For this review, take the finished solid that the model builds, in its own axes (mm). Face numbers are marked on the shaded views. Give positions to 0.01 mm unless a question says otherwise; leave off trailing zeros. Write each loop counter-clockwise with the first axis right and the second up, starting at its lowest first coordinate (ties: lowest second). Pieces come first, ordered by that corner, then holes.
from build123d import *

# Parameters (mm, degrees)
SKETCH_1_W               = 4
SKETCH_1_H               = 2.4
SKETCH_2_OUTSIDE_W       = 12.314
SKETCH_2_OUTSIDE_H       = 12.314
CUT_EXTRUDE_1_DEPTH      = 2.4
SKETCH_3_R               = 1.5
CUT_EXTRUDE_2_DEPTH      = 1
CUT_EXTRUDE_2_DEPTH_BACK = 3.4
CHAMFER_1_SIZE           = 0.4


with BuildPart() as part:
    # Эскиз1 → Повернуть1 (revolve)
    with BuildSketch(Plane(origin=(0, 0, 0), x_dir=(1, 0, 0), z_dir=(0, 1, 0))):
        with Locations((-2, 1.2)):
            Rectangle(SKETCH_1_W, SKETCH_1_H)
    revolve(axis=Axis((0, 0, 0), (0, 0, -1)))

    # Эскиз2 outside → Вырез-Вытянуть1 (cut)
    with BuildSketch(Plane.XY):
        Rectangle(SKETCH_2_OUTSIDE_W, SKETCH_2_OUTSIDE_H)
        Polygon((2.75, -1.58771324), (2.75, 1.58771324), (0, 3.175426481), (-2.75, 1.58771324), (-2.75, -1.58771324), (0, -3.175426481), align=None, mode=Mode.SUBTRACT)
    extrude(amount=-CUT_EXTRUDE_1_DEPTH, mode=Mode.SUBTRACT)

    # Эскиз3 → Вырез-Вытянуть2 (cut, two sides)
    with BuildSketch(Plane.XY) as cut_extrude_2_sk:
        Circle(SKETCH_3_R)
    extrude(amount=CUT_EXTRUDE_2_DEPTH, mode=Mode.SUBTRACT)
    extrude(cut_extrude_2_sk.sketch, amount=-CUT_EXTRUDE_2_DEPTH_BACK, mode=Mode.SUBTRACT)

    # Эскиз4 → Вырез-Повернуть1 (revolve, cut)
    with BuildSketch(Plane(origin=(0, 0, 0), x_dir=(0, 0, -1), z_dir=(1, 0, 0))):
        Polygon((0, 2.6), (0.332222633, 3.175426481), (0, 3.175426481), align=None)
        Polygon((2.4, 2.6), (2.067777367, 3.175426481), (2.4, 3.175426481), align=None)
    revolve(axis=Axis((0, 0, 0), (0, 0, -1)), mode=Mode.SUBTRACT)

    # Фаска1
    chamfer_1_edges = [part.edges().sort_by_distance(p)[0] for p in [
        (-1.5, 0, -2.4),
        (-1.5, 0, 0),
    ]]
    chamfer(chamfer_1_edges, length=CHAMFER_1_SIZE)


solid = part.part
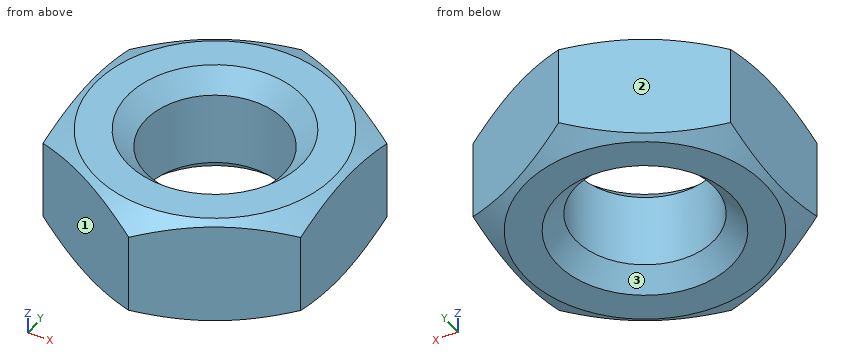
(1) Clearance check with a flat-ended pin moving along its axis: pin 1 Ø1.5 at (x, y) = (-2, -1.5) entering from +Z. State where the tip first meets the part, or that it passes through.
(2) The part is to be moulded in two halves that separate along Y. For the marked faces 1, 2 and 3, say which applies: +Y half, -Y half, draft (parallel to the pull), parting line (faces both ways), or undercut.
(3) We need section A-A (y = 0). Write out the cut boundary in (x, z), and give its area (3 significant figures).
(4) We need section C-C (z = -0.2). Write out the cut boundary in (x, y), and give its area (3 significant figures).
(5) For L1, parallel to Z at x = -0.05, y = 2.75; L2, parallel to X at y = -0.5, z = -1.85; L3, parallel to X at y = 0.75, z = -1.9, list the stretches that pass through material, from the lowest coordinate up.
(6) We need section B-B (z = -0.6). Write out the cut boundary in (x, y), and give its area (3 significant figures).
The answers:
1. pin 1: stops at z = 0
2. face 1: -Y half
2. face 2: +Y half
2. face 3: undercut
3. outline: (-2.75, -2.31) - (-2.6, -2.4) - (-1.9, -2.4) - (-1.5, -2) - (-1.5, -0.4) - (-1.9, 0) - (-2.6, 0) - (-2.75, -0.09) - close; (1.5, -2) - (1.9, -2.4) - (2.6, -2.4) - (2.75, -2.31) - (2.75, -0.09) - (2.6, 0) - (1.9, 0) - (1.5, -0.4) - close
3. area: 5.65 mm2
4. outline: (-2.75, -1.06) arc R2.95 ccw to (-2.29, -1.85) - (-0.46, -2.91) arc R2.95 ccw to (0.46, -2.91) - (2.29, -1.85) arc R2.95 ccw to (2.75, -1.06) - (2.75, 1.06) arc R2.95 ccw to (2.29, 1.85) - (0.46, 2.91) arc R2.95 ccw to (-0.46, 2.91) - (-2.29, 1.85) arc R2.95 ccw to (-2.75, 1.06) - close; hole circle Ø3.4 at (0, 0)
4. area: 16.5 mm2
5. L1: z = -2.31 to -0.09
5. L2: x = -2.75 to -1.41, 1.41 to 2.75
5. L3: x = -2.75 to -1.3, 1.3 to 2.75
6. outline: (-2.75, -1.59) - (0, -3.18) - (2.75, -1.59) - (2.75, 1.59) - (0, 3.18) - (-2.75, 1.59) - close; hole circle Ø3 at (0, 0)
6. area: 19.1 mm2
